```python
from build123d import *

# Parameters (mm, degrees)
F1_DEPTH = 101.6
F3_DEPTH = 32.8108554164


with BuildPart() as f1:
    # F0 (on Right) → F1 (new body)
    with BuildSketch(Plane.YZ):
        with BuildLine():
            Line((-15.6854130328, 37.9903614521), (-15.6854130328, -9.2097846791))
            Line((-15.6854130328, -9.2097846791), (17.1244423836, -9.2097846791))
            Line((17.1244423836, -9.2097846791), (17.1244423836, 37.9903614521))
            ThreePointArc((17.1244423836, 37.9903614521), (0.7195146754, 21.5854337439), (-15.6854130328, 37.9903614521))
        make_face()
        with BuildLine():
            ThreePointArc((17.1244423836, 37.9903614521), (0.7195146754, 54.3952891603), (-15.6854130328, 37.9903614521))
            Line((-15.6854130328, 37.9903614521), (-7.9286920533, 37.9903614521))
            ThreePointArc((-7.9286920533, 37.9903614521), (0.7195146754, 46.6385681808), (9.3677214042, 37.9903614521))
            Line((9.3677214042, 37.9903614521), (17.1244423836, 37.9903614521))
        make_face()
        with BuildLine():
            Line((-7.9286920533, 37.9903614521), (-15.6854130328, 37.9903614521))
            ThreePointArc((-15.6854130328, 37.9903614521), (0.7195146754, 21.5854337439), (17.1244423836, 37.9903614521))
            Line((17.1244423836, 37.9903614521), (9.3677214042, 37.9903614521))
            ThreePointArc((9.3677214042, 37.9903614521), (0.7195146754, 29.3421547234), (-7.9286920533, 37.9903614521))
        make_face()
    extrude(amount=-F1_DEPTH)

    # F2 (on face) → F3 (cut, through all)
    with BuildSketch(Plane.XZ.offset(15.6854130328)):
        Polygon((-76.2, 37.9903614521), (-76.2, -2.5324999557), (-25.4, -2.5324999557), (-25.4, 37.9903614521), (-25.4, 66.8847560883), (-76.2, 66.8847560883), align=None)
    extrude(amount=-F3_DEPTH, mode=Mode.SUBTRACT)


solid = f1.part
```
The listing builds one solid part. Answer for the finished solid, in the listing's coordinates (mm). A direction names the side the tool comes from. Round coordinates to 2 decimals unless told otherwise and drop trailing zeros. Write each loop counter-clockwise with the first axis right and the second up, starting at its lowest first coordinate (ties: lowest second). Pieces come first, ordered by that corner, then holes. Notation, with made-up numbers: (34.5, 62) -> (68.5, 62) arc R9 cw to (68.5, 66) -> close; hole circle Ø6 at (-5.5, 10). An arc over 180 degrees is marked (long way). Use CSV: the item, a comma, the result in double quotes. Start each with the question number.
(1) Section C-C on y = 5.5 is taken. Give the vertices of the cut face in (x, z), then the cut area to 3 significant figures.
(2) Section D-D on z = 35.5 is taken. Give the vertices of the cut face in (x, y).
(3) Section B-B on x = -16.5 is taken. Give the vertices of the cut face in (y, z).
(4) Consider L1, parallel to X at y = -8.5, z = 47; L2, parallel to Z at x = -61, y = -10; L3, parallel to Y at x = -14.5, z = 37. Determine where each line is inside the solid, lowest interval first. Write a range as from..to.
(5) Which of the six approach directions +Z, -Z, +X, -X, +Y, -Y give full straight-line access (tool end or side, diameter ignored) to faces 1 (the face through (0, 0, 16)), 2 (the face through (-25.4, 0, 19))?
(6) Each of these flat-tipped pins is pushed along its axis until it touches: pin 1 (5 mm diameter, centred on y = -1.5, z = 34, fed in from +X); pin 2 (4 mm diameter, centred on x = -46.5, y = 6.5, fed in from +Z); pin 3 (1.5 mm diameter, centred on x = -25, z = 42, fed in from +Y). Where does it stop, or does it pass through?
(7) Section A-A on z = 18.5 is taken. Give the vertices of the cut face in (x, y).
A:
1,outline,"(-101.6, -9.21) -> (0, -9.21) -> (0, 30.78) -> (-25.4, 30.78) -> (-25.4, -2.53) -> (-76.2, -2.53) -> (-76.2, 30.78) -> (-101.6, 30.78) -> close; (-101.6, 45.2) -> (-76.2, 45.2) -> (-76.2, 53.68) -> (-101.6, 53.68) -> close; (-25.4, 45.2) -> (0, 45.2) -> (0, 53.68) -> (-25.4, 53.68) -> close"
1,area,"2,800 mm²"
2,outline,"(-101.6, -15.69) -> (-76.2, -15.69) -> (-76.2, -7.56) -> (-101.6, -7.56) -> close; (-101.6, 9) -> (-76.2, 9) -> (-76.2, 17.12) -> (-101.6, 17.12) -> close; (-25.4, -15.69) -> (0, -15.69) -> (0, -7.56) -> (-25.4, -7.56) -> close; (-25.4, 9) -> (0, 9) -> (0, 17.12) -> (-25.4, 17.12) -> close"
3,outline,"(-15.69, -9.21) -> (17.12, -9.21) -> (17.12, 37.99) arc R16.4 ccw to (-15.69, 37.99) -> close; hole circle Ø17.3 at (0.72, 37.99)"
4,L1,"x = -101.6..-76.2, -25.4..0"
4,L2,"z = -9.21..-2.53"
4,L3,"y = -15.69..-7.87, 9.31..17.12"
5,face 1,"+Z, -Z, +X, +Y, -Y"
5,face 2,"+Z, +Y, -Y"
6,pin 1,"passes through"
6,pin 2,"stops at z = -2.53"
6,pin 3,"stops at y = 16.8"
7,outline,"(-101.6, -15.69) -> (-76.2, -15.69) -> (-76.2, 17.12) -> (-101.6, 17.12) -> close; (-25.4, -15.69) -> (0, -15.69) -> (0, 17.12) -> (-25.4, 17.12) -> close"
